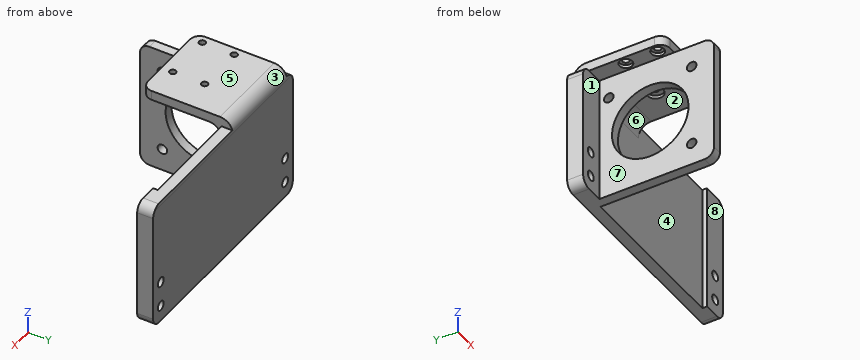
```python
from build123d import *

# Parameters (mm, degrees)
SKETCH_1_W          = 14
SKETCH_1_H          = 40
SKETCH_1_R          = 1.5
EXTRUDE_1_DEPTH     = 5
EXTRUDE_1_2_DEPTH   = 5
SKETCH_3_W          = 3
SKETCH_3_H          = 40
EXTRUDE_3_DEPTH     = 36
SKETCH_4_R          = 1.5
SKETCH_4_R_2        = 12
CUT_EXTRUDE_1_DEPTH = 30
SKETCH_8_W          = 43
SKETCH_8_H          = 5
EXTRUDE_4_DEPTH     = 40
SKETCH_9_W          = 51.8
SKETCH_9_H          = 40
CUT_EXTRUDE_2_DEPTH = 1.5
FILLET_1_R          = 3
SKETCH_10_W         = 19.3
SKETCH_10_H         = 25
SKETCH_10_R         = 1
SKETCH_10_W_2       = 5.2
SKETCH_10_H_2       = 23.5
EXTRUDE_5_DEPTH     = 3
SKETCH_11_R         = 2.5
SKETCH_11_R_2       = 2
CUT_EXTRUDE_3_DEPTH = 1
FILLET_2_R          = 4
FILLET_3_R          = 3


with BuildPart() as part:
    # Sketch 1 → Extrude 1 (new body)
    with BuildSketch(Plane(origin=(0, 0, 0), x_dir=(1, 0, 0), z_dir=(0, 1, 0))):
        with Locations((-28.5, 0)):
            Rectangle(SKETCH_1_W, SKETCH_1_H)
        with Locations(Location((-31.6, 7, 0), (0, 0, 270))):
            Circle(SKETCH_1_R, mode=Mode.SUBTRACT)
        with Locations(Location((-31.6, 15, 0), (0, 0, 270))):
            Circle(SKETCH_1_R, mode=Mode.SUBTRACT)
    extrude(amount=EXTRUDE_1_DEPTH)

    # Sketch 3 → Extrude 3 (add)
    with BuildSketch(Plane.XZ):
        with Locations((-25.8, 0)):
            Rectangle(SKETCH_3_W, SKETCH_3_H)
    extrude(amount=EXTRUDE_3_DEPTH)

    # Sketch 4 → Cut-Extrude 1 (cut)
    with BuildSketch(Plane.ZY.offset(27.3)):
        with Locations((13, -3)):
            Circle(SKETCH_4_R)
        with Locations((13, -29)):
            Circle(SKETCH_4_R)
        with Locations((-13, -29)):
            Circle(SKETCH_4_R)
        with Locations((0, -16)):
            Circle(SKETCH_4_R_2)
    extrude(amount=-CUT_EXTRUDE_1_DEPTH, mode=Mode.SUBTRACT)



with BuildPart() as body_2:
    # Sketch 1 → Extrude 1 2 (new body)
    with BuildSketch(Plane(origin=(0, 0, 0), x_dir=(1, 0, 0), z_dir=(0, 1, 0))):
        with Locations((28.5, 0)):
            Rectangle(SKETCH_1_W, SKETCH_1_H)
        with Locations(Location((31.6, 7, 0), (0, 0, 270))):
            Circle(SKETCH_1_R, mode=Mode.SUBTRACT)
        with Locations(Location((31.6, 15, 0), (0, 0, 270))):
            Circle(SKETCH_1_R, mode=Mode.SUBTRACT)
    extrude(amount=EXTRUDE_1_2_DEPTH)


with BuildPart() as part_1:
    add(part.part)

    add(body_2.part)  # Extrude 4 merges body 2
    # Sketch 8 → Extrude 4 (add)
    with BuildSketch(Plane.XY.offset(20)):
        with Locations((0, 2.5)):
            Rectangle(SKETCH_8_W, SKETCH_8_H)
    extrude(amount=-EXTRUDE_4_DEPTH)

    # Sketch 9 → Cut-Extrude 2 (cut)
    with BuildSketch(Plane.XZ):
        with Locations((1.6, 0)):
            Rectangle(SKETCH_9_W, SKETCH_9_H)
    extrude(amount=-CUT_EXTRUDE_2_DEPTH, mode=Mode.SUBTRACT)

    # Fillet 1
    fillet_1_edges = [part_1.edges().sort_by_distance(p)[0] for p in [
        (-35.5, 2.5, 20),
        (-35.5, 2.5, -20),
        (-25.8, -36, -20),
        (-25.8, -36, 20),
        (35.5, 2.5, 20),
        (35.5, 2.5, -20),
    ]]
    fillet(fillet_1_edges, radius=FILLET_1_R)

    # Sketch 10 → Extrude 5 (add)
    # profile 1 of 4: a face of its own
    with BuildSketch(Plane.XY.offset(20)):
        Polygon((-32.5, 5), (-32.5, 1.5), (-24.3, 1.5), (-5, 1.5), (-5, 5), align=None)
    # profile 2 of 4: a face of its own
    with BuildSketch(Plane.XY.offset(20)):
        with Locations((-14.65, -11)):
            Rectangle(SKETCH_10_W, SKETCH_10_H)
        with Locations((-15, -20)):
            Circle(SKETCH_10_R, mode=Mode.SUBTRACT)
        with Locations((-15, -10)):
            Circle(SKETCH_10_R, mode=Mode.SUBTRACT)
    # profile 3 of 4: a face of its own
    with BuildSketch(Plane.XY.offset(20)):
        Polygon((-32.5, 1.5), (-32.5, 0), (-27.3, 0), (-27.3, -23.5), (-24.3, -23.5), (-24.3, 1.5), align=None)
    # profile 4 of 4: a face of its own
    with BuildSketch(Plane.XY.offset(20)):
        with Locations((-29.9, -11.75)):
            Rectangle(SKETCH_10_W_2, SKETCH_10_H_2)
        with Locations((-30, -20)):
            Circle(SKETCH_10_R, mode=Mode.SUBTRACT)
        with Locations((-30, -10)):
            Circle(SKETCH_10_R, mode=Mode.SUBTRACT)
    extrude(amount=EXTRUDE_5_DEPTH)

    # Sketch 11 → Cut-Extrude 3 (cut)
    with BuildSketch(Plane(origin=(0, 0, 20), x_dir=(-1, 0, 0), z_dir=(0, 0, -1))):
        with Locations((15, -10)):
            Circle(SKETCH_11_R)
        with Locations((30, -10)):
            Circle(SKETCH_11_R_2)
        with Locations((30, -20)):
            Circle(SKETCH_11_R_2)
        with Locations((15, -20)):
            Circle(SKETCH_11_R)
    extrude(amount=-CUT_EXTRUDE_3_DEPTH, mode=Mode.SUBTRACT)

    # Fillet 2
    fillet_2_edges = [part_1.edges().sort_by_distance(p)[0] for p in [
        (-14.65, 1.5, 20),
        (-18.75, 5, 23),
    ]]
    fillet(fillet_2_edges, radius=FILLET_2_R)

    # Fillet 3
    fillet_3_edges = [part_1.edges().sort_by_distance(p)[0] for p in [
        (-5, -23.5, 21.5),
        (-32.5, -23.5, 21.5),
    ]]
    fillet(fillet_3_edges, radius=FILLET_3_R)


solid = part_1.part
```
For this review, take the finished solid that the model builds, in its own axes (mm). Face numbers are marked on the shaded views. A direction names the side the tool comes from. Give positions to 0.01 mm unless a question says otherwise; leave off trailing zeros. Write each loop counter-clockwise with the first axis right and the second up, starting at its lowest first coordinate (ties: lowest second). Pieces come first, ordered by that corner, then holes. Notation, with made-up numbers: M 78.5,84.25 L 103.5,84.25 A14 ccw 103.5,107.25 Z; hole C 61.25,79 d10. An arc over 180 degrees is marked long. Answer as CSV lines item,"result".
1. For pin 1 (1 mm diameter, centred on y = -11.5, z = 15.5, fed in from +X); pin 2 (3.5 mm diameter, centred on y = -12, z = 20.5, fed in from +X); pin 3 (4 mm diameter, centred on y = -20, z = -11.5, fed in from -X), all flat-tipped, find the tip position at first contact; note any pin that passes through.
Findings:
pin 1,"stops at x = -24.3"
pin 2,"stops at x = -5"
pin 3,"stops at x = -27.3"
2. Consider section D-D, the plane y = -16. Write out the cut boundary in (x, z).
Findings:
outline,"M -32.5,20 L -27.3,20 L -27.3,12 L -24.3,12 L -24.3,20 L -5,20 L -5,23 L -32.5,23 Z; M -27.3,-20 L -24.3,-20 L -24.3,-12 L -27.3,-12 Z"
3. Wall thickness on line 1 (X direction, y = 3, z = -15); line 2 (X direction, y = -10, z = 22); line 3 (Y direction, x = -25.5, z = 13): over which ranges is each line inside the solid? List them lowest first.
Findings:
line 1,"x = -35.5 to -33.1, -30.1 to 30.1, 33.1 to 35.5"
line 2,"x = -32.5 to -31, -29 to -16, -14 to -5"
line 3,"y = -36 to -30.5, -27.5 to -4.5, -1.5 to 5"
4. Consider section B-B, the plane z = 0. Write out the cut boundary in (x, y), then the cut area to 3 significant figures.
Findings:
outline,"M -35.5,0 L -27.3,0 L -27.3,-4 L -24.3,-4 L -24.3,1.5 L 27.5,1.5 L 27.5,0 L 35.5,0 L 35.5,5 L -35.5,5 Z; M -27.3,-36 L -24.3,-36 L -24.3,-28 L -27.3,-28 Z"
area,"313 mm2"
5. Draft analysis for pull direction X (two halves, no side actions). For the marked faces 6, 7 and 8, state which applies: +X half, -X half, draft (parallel to the pull), parting line (faces both ways), or undercut.
Findings:
face 6,"undercut"
face 7,"-X half"
face 8,"draft"
6. Consider section C-C, the plane x = -15. Write out the cut boundary in (y, z), then the cut area to 4 significant figures.
Findings:
outline,"M -23.5,20 L -22.5,20 L -22.5,21 L -21,21 L -21,23 L -23.5,23 Z; M -19,21 L -17.5,21 L -17.5,20 L -12.5,20 L -12.5,21 L -11,21 L -11,23 L -19,23 Z; M -9,21 L -7.5,21 L -7.5,20 L -2.5,20 A4 cw 1.5,16 L 1.5,-20 L 5,-20 L 5,19 A4 ccw 1,23 L -9,23 Z"
area,"207.5 mm2"
7. For the marked faces 1, 2, 3, 4 and 5, list the 3-axis set-ups (+Z, -Z, +X, -X, +Y, -Y) from which the entire face can be reached by the end or side of a thin tool; tool diameter is ignored.
Findings:
face 1,"-Z, -X, -Y"
face 2,"-Z, +X, -Y"
face 3,"+Z, +X, -X, +Y"
face 4,"-Z, -Y"
face 5,"+Z, +X, -X, +Y, -Y"
8. Consider section A-A, the plane y = -29. Write out the cut boundary in (x, z).
Findings:
outline,"M -27.3,-20 L -24.3,-20 L -24.3,-14.5 L -27.3,-14.5 Z; M -27.3,-11.5 L -24.3,-11.5 L -24.3,11.5 L -27.3,11.5 Z; M -27.3,14.5 L -24.3,14.5 L -24.3,20 L -27.3,20 Z"
